Geometry check sheet. Reference: the model listing, model coordinates, mm. Give positions to 0.01 mm unless a question says otherwise; leave off trailing zeros. Write each loop counter-clockwise with the first axis right and the second up, starting at its lowest first coordinate (ties: lowest second). Pieces come first, ordered by that corner, then holes. Notation, with made-up numbers: (-14, 56.5) - (30, 56.5) arc R7 ccw to (30, 66.5) - close; hole circle Ø4 at (-24, 2.25). An arc over 180 degrees is marked (long way). Use a Markdown table: item, result.
```python
from build123d import *

# Parameters (mm, degrees)
SKETCH_1_R      = 1.5
SKETCH_1_R_2    = 4
EXTRUDE_1_DEPTH = 3


with BuildPart() as part:
    # 草图1 → 凸台-拉伸1 (new body)
    with BuildSketch(Plane.XY):
        with BuildLine():
            Line((-2.598076211, 21.5), (-19.918584287, -8.5))
            ThreePointArc((-19.918584287, -8.5), (-19.918584287, -11.5), (-17.320508076, -13))
            Line((-17.320508076, -13), (17.320508076, -13))
            ThreePointArc((17.320508076, -13), (19.918584287, -11.5), (19.918584287, -8.5))
            Line((19.918584287, -8.5), (2.598076211, 21.5))
            ThreePointArc((2.598076211, 21.5), (0, 23), (-2.598076211, 21.5))
        make_face()
        with Locations((-17.320508076, -10)):
            Circle(SKETCH_1_R, mode=Mode.SUBTRACT)
        with Locations((0, 20)):
            Circle(SKETCH_1_R, mode=Mode.SUBTRACT)
        with Locations((17.320508076, -10)):
            Circle(SKETCH_1_R, mode=Mode.SUBTRACT)
        Circle(SKETCH_1_R_2, mode=Mode.SUBTRACT)
        with Locations((0, 6.5)):
            Circle(SKETCH_1_R, mode=Mode.SUBTRACT)
        with Locations((0, -6.5)):
            Circle(SKETCH_1_R, mode=Mode.SUBTRACT)
    extrude(amount=EXTRUDE_1_DEPTH)


solid = part.part
```
1) Section check A-A on y = -10. Record the boundary of the cut face in (x, z), then the cut area to 3 significant figures.
Working result:
| item | result |
|---|---|
| outline | (-20.32, 0) - (-18.82, 0) - (-18.82, 3) - (-20.32, 3) - close; (-15.82, 0) - (15.82, 0) - (15.82, 3) - (-15.82, 3) - close; (18.82, 0) - (20.32, 0) - (20.32, 3) - (18.82, 3) - close |
| area | 104 mm² |
2) Depth check by flat-ended pin: P1, Ø3.5, axis at x = -17.32, y = -10, coming from the +Z side; P2, Ø2.5, axis at x = 0, y = -6.5, coming from the +Z side; P3, Ø1, axis at x = -2.5, z = 2.5, coming from the +Y side. Enter the tip coordinate at first touch or a pass-through.
Working result:
| item | result |
|---|---|
| P1 | stops at z = 3 |
| P2 | passes through |
| P3 | stops at y = 22.24 |
3) Section check B-B on z = 0.45. Record the boundary of the cut face in (x, y), then the cut area to 3 significant figures.
Working result:
| item | result |
|---|---|
| outline | (-19.92, -8.5) arc R3 ccw to (-17.32, -13) - (17.32, -13) arc R3 ccw to (19.92, -8.5) - (2.6, 21.5) arc R3 ccw to (-2.6, 21.5) - close; hole circle Ø3 at (-17.32, -10); hole circle Ø8 at (0, 0); hole circle Ø3 at (0, -6.5); hole circle Ø3 at (0, 6.5); hole circle Ø3 at (0, 20); hole circle Ø3 at (17.32, -10) |
| area | 774 mm² |
4) Mould release check, pull along X, two halves, no side actions. Record for faces 1 (the cylindrical face through (0, -8, 1)), 2 (the cylindrical face through (0, 23, 1)), 3 (the cylindrical face through (-0.867, -3.905, 1.479)), 4 (the flat face through (11.38, 6.29, 1.48)): pulls with the +X half, pulls with the -X half, needs draft (parallel to the pull), parting line crosses it, or undercut.
Working result:
| item | result |
|---|---|
| face 1 | undercut |
| face 2 | parting line crosses it |
| face 3 | undercut |
| face 4 | pulls with the +X half |
5) Section check D-D on y = 7. Record the boundary of the cut face in (x, z), then the cut area to 3 significant figures.
Working result:
| item | result |
|---|---|
| outline | (-10.97, 0) - (-1.41, 0) - (-1.41, 3) - (-10.97, 3) - close; (1.41, 0) - (10.97, 0) - (10.97, 3) - (1.41, 3) - close |
| area | 57.3 mm² |
6) Material ranges on L1, parallel to Y at x = 0, z = 2.35; L2, parallel to Y at x = 2.5, z = 0.95; L3, parallel to X at y = 7.5, z = 2.05, recorded low to high. Write a range as from..to.
Working result:
| item | result |
|---|---|
| L1 | y = -13..-8, -5..-4, 4..5, 8..18.5, 21.5..23 |
| L2 | y = -13..-3.12, 3.12..21.66 |
| L3 | x = -10.68..-1.12, 1.12..10.68 |
7) Section check C-C on x = 16.5. Record the boundary of the cut face in (y, z).
Working result:
| item | result |
|---|---|
| outline | (-13, 0) - (-11.26, 0) - (-11.26, 3) - (-13, 3) - close; (-8.74, 0) - (-2.58, 0) - (-2.58, 3) - (-8.74, 3) - close |
